from build123d import *

# Parameters (mm, degrees)
SKETCH_2_R          = 14
EXTRUDE_1_DEPTH     = 8
SKETCH_3_R          = 8.5
EXTRUDE_2_DEPTH     = 20
SKETCH_4_R          = 5
CUT_EXTRUDE_1_DEPTH = 45
EXTRUDE_START       = -7
SKETCH_5_R          = 5
SKETCH_5_R_2        = 2.75
EXTRUDE_3_DEPTH     = 7
CUT_EXTRUDE_START   = -3.3
SKETCH_6_R          = 5
SKETCH_6_R_2        = 2.75
CUT_EXTRUDE_2_DEPTH = 3.3
EXTRUDE_4_DEPTH     = 6
SKETCH_9_R          = 6
CUT_EXTRUDE_5_DEPTH = 21
CHAMFER_5_SIZE      = 0.5
SKETCH_21_R         = 25
EXTRUDE_5_DEPTH     = 3
SKETCH_22_R         = 2
SKETCH_22_R_2       = 25
CUT_EXTRUDE_7_DEPTH = 3
FILLET_2_R          = 3
FILLET_3_R          = 0.5
SKETCH_23_R         = 6
CUT_EXTRUDE_8_DEPTH = 3
CHAMFER_7_SIZE      = 0.5
EXTRUDE_6_DEPTH     = 6
CHAMFER_8_SIZE      = 0.5


with BuildPart() as part:
    # Sketch 2 → Extrude 1 (new body)
    with BuildSketch(Plane(origin=(0, 0, 0), x_dir=(1, 0, 0), z_dir=(0, 1, 0))):
        with Locations(Location((0, 0, 0), (0, 0, 270))):
            Circle(SKETCH_2_R)
    extrude(amount=EXTRUDE_1_DEPTH)

    # Sketch 3 → Extrude 2 (add)
    with BuildSketch(Plane(origin=(0, 8, 0), x_dir=(1, 0, 0), z_dir=(0, 1, 0))):
        with Locations(Location((0, 0, 0), (0, 0, 270))):
            Circle(SKETCH_3_R)
    extrude(amount=EXTRUDE_2_DEPTH)

    # Sketch 4 → Cut-Extrude 1 (cut)
    with BuildSketch(Plane.XZ):
        with Locations(Location((0, 0, 0), (0, 0, 270))):
            Circle(SKETCH_4_R)
    extrude(amount=-CUT_EXTRUDE_1_DEPTH, mode=Mode.SUBTRACT)

    # Sketch 5 → Extrude 3 (add)
    with BuildSketch(Plane(origin=(0, 28, 0), x_dir=(1, 0, 0), z_dir=(0, 1, 0)).offset(EXTRUDE_START)):
        with Locations(Location((0, 0, 0), (0, 0, 90))):
            Circle(SKETCH_5_R)
        with Locations(Location((0, 0, 0), (0, 0, 270))):
            Circle(SKETCH_5_R_2, mode=Mode.SUBTRACT)
    extrude(amount=EXTRUDE_3_DEPTH)

    # Sketch 6 → Cut-Extrude 2 (cut)
    with BuildSketch(Plane(origin=(0, 28, 0), x_dir=(1, 0, 0), z_dir=(0, 1, 0)).offset(CUT_EXTRUDE_START)):
        with Locations(Location((0, 0, 0), (0, 0, 90))):
            Circle(SKETCH_6_R)
        with Locations(Location((0, 0, 0), (0, 0, 270))):
            Circle(SKETCH_6_R_2, mode=Mode.SUBTRACT)
    extrude(amount=CUT_EXTRUDE_2_DEPTH, mode=Mode.SUBTRACT)

    # Sketch 8 → Extrude 4 (add)
    with BuildSketch(Plane(origin=(0, 28, 0), x_dir=(1, 0, 0), z_dir=(0, 1, 0))):
        with BuildLine():
            Line((-3, 4), (-7.5, 4))
            ThreePointArc((-7.5, 4), (0, -8.5), (7.5, 4))
            Line((7.5, 4), (3, 4))
            ThreePointArc((3, 4), (0, -5), (-3, 4))
        make_face()
    extrude(amount=EXTRUDE_4_DEPTH)

    # Sketch 9 → Cut-Extrude 5 (cut)
    with BuildSketch(Plane.XZ):
        with Locations(Location((0, 0, 0), (0, 0, 270))):
            Circle(SKETCH_9_R)
    extrude(amount=-CUT_EXTRUDE_5_DEPTH, mode=Mode.SUBTRACT)

    # Chamfer 5
    chamfer_5_edges = [part.edges().sort_by_distance(p)[0] for p in [
        (0, 8, -14),
    ]]
    chamfer(chamfer_5_edges, length=CHAMFER_5_SIZE)

    # Sketch 21 → Extrude 5 (add)
    with BuildSketch(Plane.XZ):
        with Locations(Location((0, 0, 0), (0, 0, 270))):
            Circle(SKETCH_21_R)
    extrude(amount=EXTRUDE_5_DEPTH)

    # Sketch 22 → Cut-Extrude 7 (cut)
    with BuildSketch(Plane.XZ.offset(3)):
        with Locations(Location((0, 20, 0), (0, 0, 270))):
            Circle(SKETCH_22_R)
        with Locations((0, -40)):
            Circle(SKETCH_22_R_2)
        with Locations(Location((17.320508076, -10, 0), (0, 0, 270))):
            Circle(SKETCH_22_R)
        with Locations((-34.641016151, 20)):
            Circle(SKETCH_22_R_2)
        with Locations(Location((-17.320508076, -10, 0), (0, 0, 270))):
            Circle(SKETCH_22_R)
        with Locations((34.641016151, 20)):
            Circle(SKETCH_22_R_2)
    extrude(amount=-CUT_EXTRUDE_7_DEPTH, mode=Mode.SUBTRACT)

    # Fillet 2
    fillet_2_edges = [part.edges().sort_by_distance(p)[0] for p in [
        (-24.820508076, -1.5, -2.990381057),
        (-9.820508076, -1.5, 22.990381057),
        (9.820508076, -1.5, 22.990381057),
        (24.820508076, -1.5, -2.990381057),
        (15, -1.5, -20),
        (-15, -1.5, -20),
    ]]
    fillet(fillet_2_edges, radius=FILLET_2_R)

    # Fillet 3
    fillet_3_edges = [part.edges().sort_by_distance(p)[0] for p in [
        (0, 0, -14),
    ]]
    fillet(fillet_3_edges, radius=FILLET_3_R)

    # Sketch 23 → Cut-Extrude 8 (cut)
    with BuildSketch(Plane.XZ.offset(3)):
        with Locations(Location((0, 0, 0), (0, 0, 270))):
            Circle(SKETCH_23_R)
    extrude(amount=-CUT_EXTRUDE_8_DEPTH, mode=Mode.SUBTRACT)

    # Chamfer 7
    chamfer_7_edges = [part.edges().sort_by_distance(p)[0] for p in [
        (0, -3, 6),
    ]]
    chamfer(chamfer_7_edges, length=CHAMFER_7_SIZE)

    # Sketch 24 → Extrude 6 (add)
    with BuildSketch(Plane(origin=(0, 34, 0), x_dir=(1, 0, 0), z_dir=(0, 1, 0))):
        with BuildLine():
            Line((-7.5, 4), (-3, 4))
            ThreePointArc((-3, 4), (0, -5), (3, 4))
            Line((3, 4), (7.5, 4))
            ThreePointArc((7.5, 4), (0, -8.5), (-7.5, 4))
        make_face()
    extrude(amount=EXTRUDE_6_DEPTH)

    # Chamfer 8
    chamfer_8_edges = [part.edges().sort_by_distance(p)[0] for p in [
        (0, 40, 8.5),
    ]]
    chamfer(chamfer_8_edges, length=CHAMFER_8_SIZE)


solid = part.part
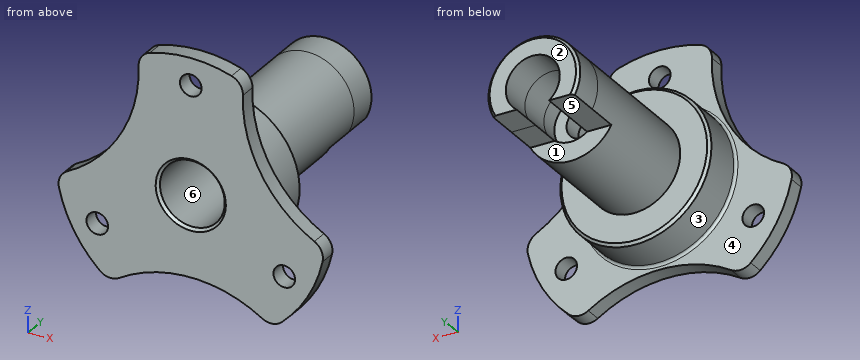
Work out the finished part from the listing and answer in its coordinate system (mm). Face numbers are marked on the shaded views. A direction names the side the tool comes from. Round coordinates to 2 decimals unless told otherwise and drop trailing zeros. Order: outer loops, then holes, each group sorted by start corner. A loop starts at its lowest first (then second) coordinate and runs counter-clockwise, first axis right, second up. Notation, with made-up numbers: M 87,22.25 L 131,22.25 A17 cw 131,29.25 Z; hole C 14,21.5 d2. An arc over 180 degrees is marked long. One line per item, written item: value.
Q1. Find section D-D on z = -10. Give the number of separate pieces and of enclosed holes in the cut face, then the cut area to 3 significant figures.
Derived:
separate pieces: 3
enclosed holes: 0
area: 270 mm²
Q2. Find section C-C on y = 33. Write down the section's boundary in (x, z).
Derived:
outline: M -7.5,-4 L -3,-4 A5 cw long 3,-4 L 7.5,-4 A8.5 ccw long Z
Q3. Find section A-A on z = 20. Write down the section's boundary in (x, y), then the cut area to 3 significant figures.
Derived:
outline: M -9.64,-3 L -2,-3 L -2,0 L -9.64,0 Z; M 2,-3 L 9.64,-3 L 9.64,0 L 2,0 Z
area: 45.8 mm²
Q4. Flat-ended cylindrical pins translate along their axes: pin 1 (5 mm diameter, centred on x = -17.32, z = -10, fed in from -Y); pin 2 (1.5 mm diameter, centred on y = 33, z = -5, fed in from +X); pin 3 (8 mm diameter, centred on x = -3.5, z = -14.5, fed in from +Y); pin 4 (5 mm diameter, centred on x = 5.5, y = 38, fed in from -Z). Find the tip coordinate at first contact, or state that the pin passes through.
Derived:
pin 1: y = -3
pin 2: through
pin 3: y = 8
pin 4: z = -4
Q5. Determine the mould class of the marked faces 4, 5 and 6 for opening direction Z: released by +Z, released by -Z, zero draft, split by the parting line, or undercut.
Derived:
face 4: zero draft
face 5: released by -Z
face 6: undercut
Q6. For the marked faces 1, 2 and 3, determine the directions among +Z, -Z, +X, -X, +Y, -Y from which every point of the face is accessible in a straight line to the end or side of a thin tool.
Derived:
face 1: -Z, +X, -X, +Y
face 2: +Z, -Z, +X, -X, +Y
face 3: +Y
Q7. Straight lines are drawn through the part: line 1 (X direction, y = 3, z = 0); line 2 (Z direction, x = -4, y = 27.5); line 3 (Y direction, x = 8.5, z = 6). For each, find the intervals that lie inside material, in ascending order.
Derived:
line 1: -14 to -6, 6 to 14
line 2: -7.5 to -3, 3 to 7.5
line 3: -3 to 8
Q8. Find section B-B on y = 4. Write down the section's boundary in (x, z), then the cut area to 3 significant figures.
Derived:
outline: C 0,0 d28; hole C 0,0 d12
area: 503 mm²
